The listing builds one solid part. Answer for the finished solid, in the listing's coordinates (mm). A direction names the side the tool comes from. Give positions to 0.01 mm unless a question says otherwise; leave off trailing zeros. Loops run counter-clockwise (first coordinate to the right, second up) from the corner with the lowest first, then second, coordinate; pieces in that order, holes last. Notation, with made-up numbers: (87.5, -30.75) - (118.5, -30.75) arc R26 cw to (118.5, -5.75) - close; hole circle Ø8 at (23.25, 55). An arc over 180 degrees is marked (long way). Answer in a Markdown table with one row per item. Add a question column.
```python
from build123d import *

# Parameters (mm, degrees)
SKETCH2_R = 3.5


with BuildPart() as part:
    # Sketch1 → Revolve1 (revolve)
    with BuildSketch(Plane.XY, mode=Mode.PRIVATE) as revolve1_sk:
        Polygon((-170, 0), (-170, 20), (-150, 20), (-150, 12.5), (-110, 12.5), (-110, 30), (-60, 30), (-60, 17.5), (-30, 17.5), (-30, 45), (0, 45), (0, 0), align=None)
    revolve1 = revolve(revolve1_sk.sketch.rotate(Axis((-99.144385027, 0, 0), (1, 0, 0)), 90), axis=Axis((-99.144385027, 0, 0), (1, 0, 0)))

    # Sketch2 → Cut-Revolve1 (revolve, cut)
    with BuildSketch(Plane.XY, mode=Mode.PRIVATE) as cut_revolve1_sk:
        with Locations((-160, 20.12160323)):
            Circle(SKETCH2_R)
    revolve(cut_revolve1_sk.sketch.rotate(Axis((-170, 0, 0), (1, 0, 0)), 90), axis=Axis((-170, 0, 0), (1, 0, 0)), mode=Mode.SUBTRACT)

    # Mirror1: Revolve1 across plane
    add(revolve1.mirror(Plane(origin=(0, 0, 0), x_dir=(0, 0, 1), z_dir=(1, 0, 0))))


solid = part.part
```
(1) A cutting plane is placed at C-C on z = -34.5. Determine the outline of the cut face in (x, y).
(2) The mould has two halves that part along X. Classify faces 5 (the face through (-153.21, -0.88, -19.98)), 6 (the face through (170, 0, 0)), 7 (the face through (-150, -9, 9)): pulls with the +X half, pulls with the -X half, needs draft (parallel to the pull), parting line crosses it, or undercut.
(3) A cutting plane is placed at B-B on x = -7. Determine the outline of the cut face in (y, z).
(4) A cutting plane is placed at A-A on y = -25. Determine the outline of the cut face in (x, z), plus the area to 3 significant figures.
(5) A tool of negligible diameter and unlimited length cuts with its end or side. For faces 1 (the face through (-30, 19, 1)), 2 (the face through (-84.65, -25.296, 16.128)), 3 (the face through (84.65, -25.296, 16.128)), 4 (the face through (-170, 0, 0)), from which of +Z, -Z, +X, -X, +Y, -Y can it reach the whole face along a straight path? Write none if from no direction.
(6) A cutting plane is placed at D-D on x = 120. Determine the outline of the cut face in (y, z).
(7) Find the intervals of material crossed by line 1 along X through (y, z) = (9.5, 23); line 2 along X through (y, z) = (-3, 15.5); line 3 along X through (y, z) = (17, -8), in increasing order. Write a range as [from, to].
(8) Given pin 1 Ø1 at (x, z) = (-97.5, 17) entering from +Y; pin 2 Ø2 at (x, y) = (114, -4) entering from +Z; pin 3 Ø1 at (x, z) = (78.5, 22.5) entering from -Y, each flat-ended and moving along its own axis, determine where each tip first touches the part or whether it passes through.
Evaluation:
| question | item | result |
|---|---|---|
| 1 | outline | (-30, -28.89) - (30, -28.89) - (30, 28.89) - (-30, 28.89) - close |
| 2 | face 5 | needs draft |
| 2 | face 6 | pulls with the +X half |
| 2 | face 7 | undercut |
| 3 | outline | circle Ø90 at (0, 0) |
| 4 | outline | (-110, -16.58) - (-60, -16.58) - (-60, 16.58) - (-110, 16.58) - close; (-30, -37.42) - (30, -37.42) - (30, 37.42) - (-30, 37.42) - close; (60, -16.58) - (110, -16.58) - (110, 16.58) - (60, 16.58) - close |
| 4 | area | 7,810 mm² |
| 5 | face 1 | none |
| 5 | face 2 | -X |
| 5 | face 3 | +X |
| 5 | face 4 | +Z, -Z, -X, +Y, -Y |
| 6 | outline | circle Ø25 at (0, 0) |
| 7 | line 1 | x = [-110, -60], [-30, 30], [60, 110] |
| 7 | line 2 | x = [-170, -150], [-110, 110], [150, 170] |
| 7 | line 3 | x = [-170, -163.24], [-156.76, -150], [-110, -60], [-30, 30], [60, 110], [150, 170] |
| 8 | pin 1 | stops at y = 25.05 |
| 8 | pin 2 | stops at z = 12.13 |
| 8 | pin 3 | stops at y = -20.4 |
